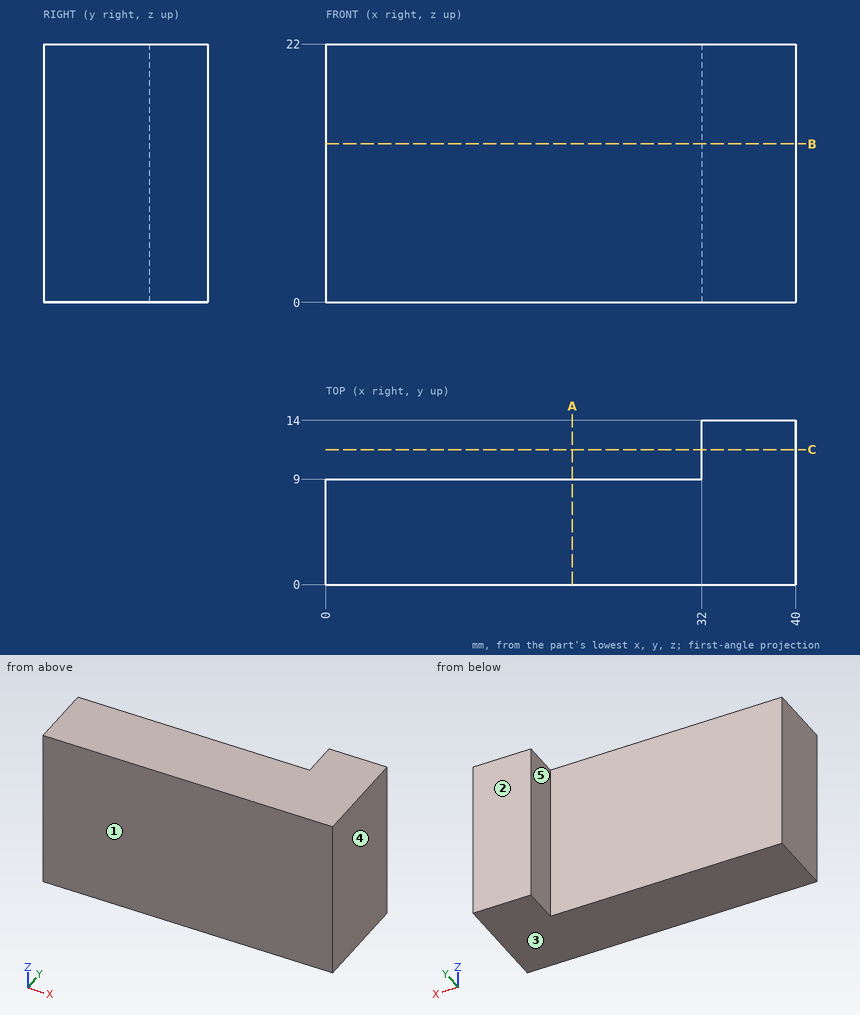
Job drawing, mm, ordinate dimensions from the low corner. One solid piece. A direction names the side the tool comes from. Give positions to 0.01 mm unless a question says otherwise; leave off trailing zeros. Order: outer loops, then holes, each group sorted by start corner. A loop starts at its lowest first (then second) coordinate and runs counter-clockwise, first axis right, second up. Notation, with made-up numbers: (88, -22.5) - (99, -22.5) arc R16 cw to (99, -13.5) - close; hole circle Ø8 at (59.25, 51.25). An arc over 180 degrees is marked (long way). Answer in a Markdown table with one row per item.
1. Saw through at B-B, the plane z = 13.5. Give the cut face in (x, y), plus the area to 3 significant figures.
Data:
| item | result |
|---|---|
| outline | (0, 0) - (40, 0) - (40, 14) - (32, 14) - (32, 9) - (0, 9) - close |
| area | 400 mm² |
2. Probe probe 1 along X at (y, z) = (12.75, 18); probe 2 along Y at (x, z) = (5.5, 14.25). List the from-to ranges inside material, lowest first. Write a range as [from, to].
Data:
| item | result |
|---|---|
| probe 1 | x = [32, 40] |
| probe 2 | y = [0, 9] |
3. Tool access for the marked faces 4 and 5: list every direction of +Z, -Z, +X, -X, +Y, -Y with a clear straight run to the whole face (end or side of a thin tool).
Data:
| item | result |
|---|---|
| face 4 | +Z, -Z, +X, +Y, -Y |
| face 5 | +Z, -Z, -X, +Y |
4. Flat gauge pins, fed straight in: pin 1 (6 mm diameter, centred on x = 20.5, z = 10, fed in from +Y); pin 2 (1.5 mm diameter, centred on x = 23.5, y = 10, fed in from -Z). Where does each tip first touch, or does it go through?
Data:
| item | result |
|---|---|
| pin 1 | stops at y = 9 |
| pin 2 | passes through |
5. Pull direction Y, two halves, no side cores. Call the marked faces 1, 2 and 3: pulls with the +Y half, pulls with the -Y half, needs draft (parallel to the pull), parting line crosses it, or undercut.
Data:
| item | result |
|---|---|
| face 1 | pulls with the -Y half |
| face 2 | pulls with the +Y half |
| face 3 | needs draft |
6. Saw through at A-A, the plane x = 21. Give the cut face in (y, z).
Data:
| item | result |
|---|---|
| outline | (0, 0) - (9, 0) - (9, 22) - (0, 22) - close |
7. Saw through at C-C, the plane y = 11.5. Give the cut face in (x, z), plus the area to 3 significant figures.
Data:
| item | result |
|---|---|
| outline | (32, 0) - (40, 0) - (40, 22) - (32, 22) - close |
| area | 176 mm² |
